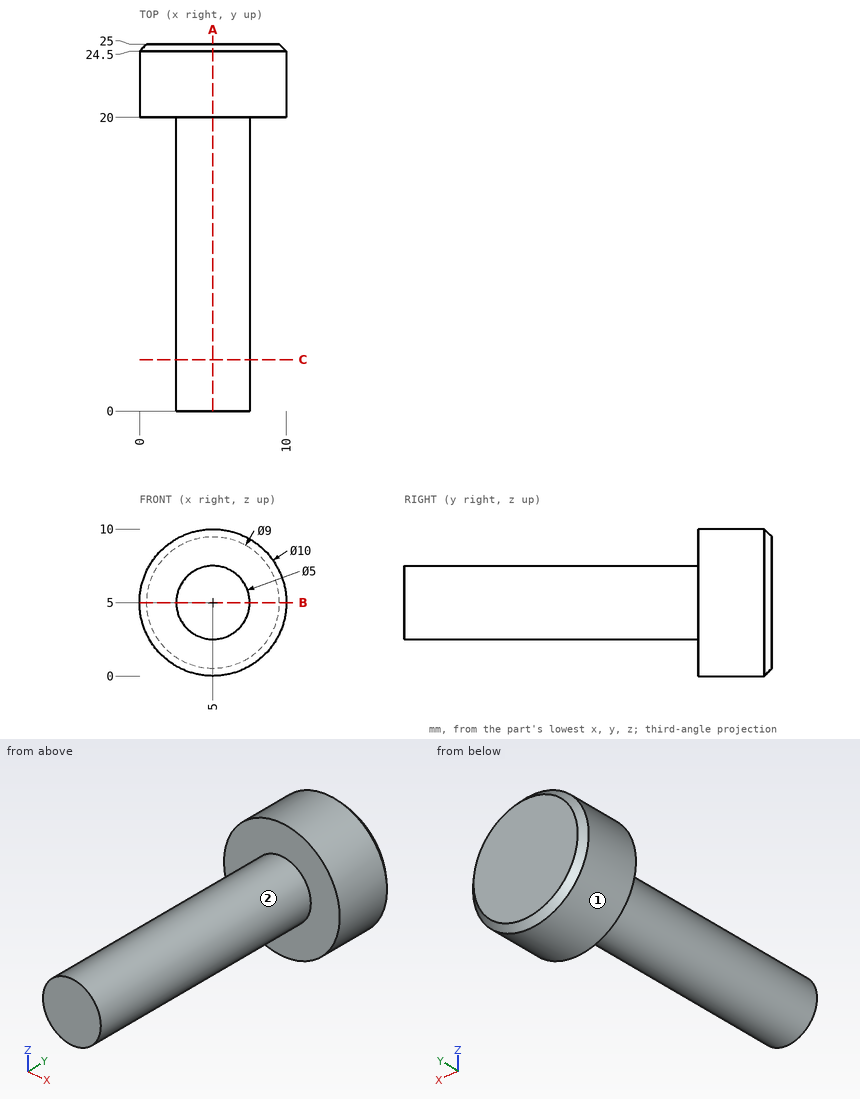
Here's the drawing with two shaded views (mm, measured from the low corner). I have some questions. A direction names the side the tool comes from. Coordinates: 2 decimals unless noted, no trailing zeros. Loops run counter-clockwise (first coordinate to the right, second up) from the corner with the lowest first, then second, coordinate; pieces in that order, holes last. Notation, with made-up numbers: M 85.5,88.25 L 120.5,88.25 A25 cw 120.5,119.25 Z; hole C 80.5,42.25 d5. An arc over 180 degrees is marked long. Answer as CSV lines item,"result". Start each with the question number.
1. Suppose I cut it at C-C, the plane y = 3.5. List the corners of the cut face in (x, z) for me.
2. Suppose I cut it at A-A, the plane x = 5. List the corners of the cut face in (y, z) for me, plus the area to 3 significant figures.
3. For the marked faces 1 and 2, which set-ups out of +Z, -Z, +X, -X, +Y, -Y let a thin tool reach every point of the face, with its end or its side?
4. If I drill on probe 1 along Y at (x, z) = (7, 7.25); probe 2 along Z at (x, y) = (5, 17); probe 3 along X at (y, z) = (13.75, 7), over which ranges is the centre line in solid material (lowest first)? Write a range as [from, to].
5. For pin 1 Ø1 at (y, z) = (7, 3.5) entering from +X; pin 2 Ø3 at (x, y) = (6.5, 15) entering from -Z; pin 3 Ø4 at (y, z) = (7, 6.5) entering from -X; pin 4 Ø3 at (x, z) = (8, 4) entering from -Y, each with a flat end and sliding along its axis, tell me the tip position at first contact or that it passes through.
6. Suppose I cut it at B-B, the plane z = 5. List the corners of the cut face in (x, y) for me.
Output:
1,outline,"C 5,5 d5"
2,outline,"M 0,2.5 L 20,2.5 L 20,0 L 24.5,0 L 25,0.5 L 25,9.5 L 24.5,10 L 20,10 L 20,7.5 L 0,7.5 Z"
2,area,"150 mm^2"
3,face 1,"+Y, -Y"
3,face 2,"-Y"
4,probe 1,"y = [20, 25]"
4,probe 2,"z = [2.5, 7.5]"
4,probe 3,"x = [3.5, 6.5]"
5,pin 1,"stops at x = 7.29"
5,pin 2,"stops at z = 2.5"
5,pin 3,"stops at x = 2.5"
5,pin 4,"stops at y = 0"
6,outline,"M 0,20 L 2.5,20 L 2.5,0 L 7.5,0 L 7.5,20 L 10,20 L 10,24.5 L 9.5,25 L 0.5,25 L 0,24.5 Z"
